Check sheet for the drawn part. Datum: minimum x, y, z corner. Units: mm. Round coordinates to 2 decimals unless told otherwise and drop trailing zeros. Loops run counter-clockwise (first coordinate to the right, second up) from the corner with the lowest first, then second, coordinate; pieces in that order, holes last. Notation, with made-up numbers: (46, 65.25) -> (105, 65.25) arc R8 cw to (105, 72.25) -> close; hole circle Ø11 at (20.5, 65.25). An arc over 180 degrees is marked (long way). Write item = value, one per line. Start each with the question number.
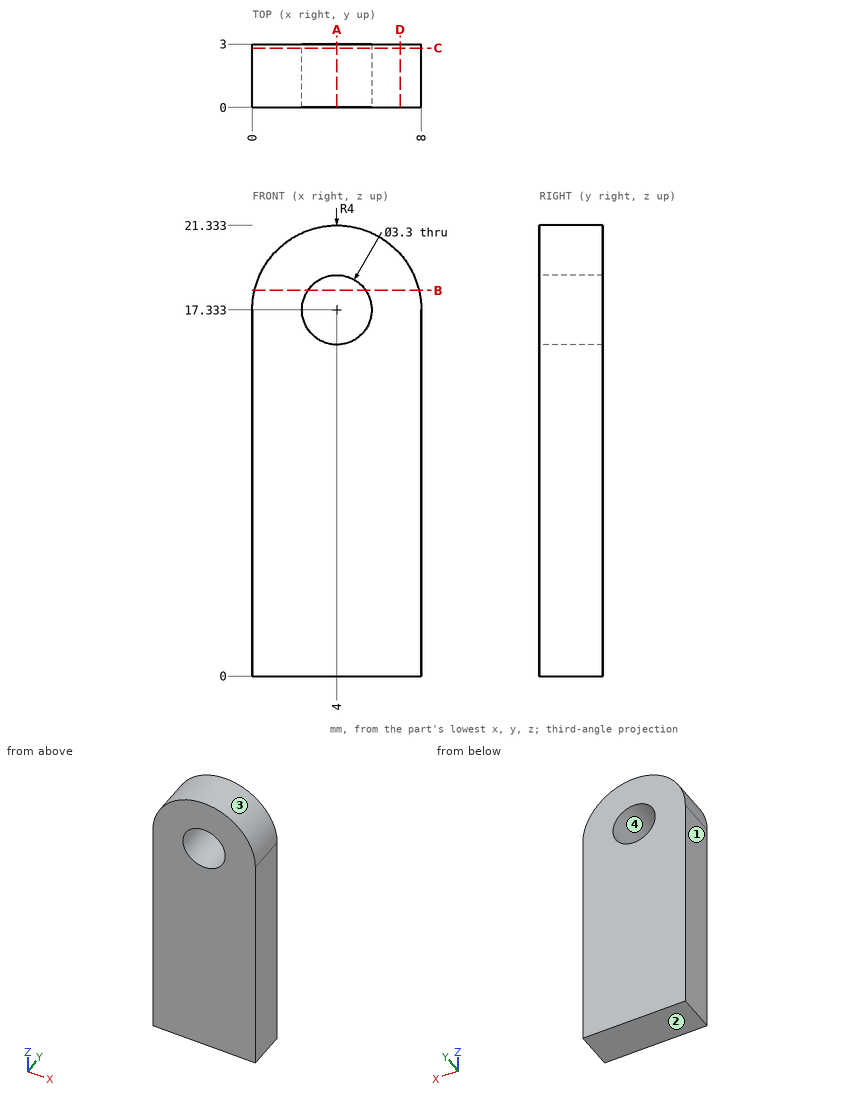
(1) Draft check along Z on the marked faces 1, 2, 3 and 4. Enter one of: +Z half, -Z half, draft (parallel to the pull), parting line (faces both ways), or undercut.
(2) Section check C-C on y = 2.8. Enter the section's corners in (x, z).
(3) Scan lines: line 1 (Z direction, x = 4, y = 2); line 2 (Z direction, x = 5, y = 2.8) (1 decimal); line 3 (X direction, y = 2.65, z = 16.5). Record each from-to range of solid material in increasing order. Write a range as [from, to].
(4) Depth check by flat-ended pin: pin 1 Ø1.5 at (x, y) = (3, 2.5) entering from +Z (3 decimals); pin 2 Ø2 at (x, z) = (6, 4.5) entering from -Y; pin 3 Ø1 at (x, y) = (7, 0.5) entering from +Z; pin 4 Ø3 at (x, z) = (4, 17.33) entering from +Y. Enter the tip coordinate at first touch or a pass-through.
(5) Section check D-D on x = 7. Enter the section's corners in (y, z).
(6) Section check B-B on z = 18.25. Enter the section's corners in (x, y).
(7) Section check A-A on x = 4. Enter the section's corners in (y, z), then the cut area to 3 significant figures.
Computed values:
q1.face_1 = draft
q1.face_2 = -Z half
q1.face_3 = +Z half
q1.face_4 = undercut
q2.outline = (0, 0) -> (8, 0) -> (8, 17.33) arc R4 ccw to (0, 17.33) -> close; hole circle Ø3.3 at (4, 17.33)
q3.line_1 = [0, 15.68], [18.98, 21.33]
q3.line_2 = [0, 16], [18.6, 21.2]
q3.line_3 = [0, 2.58], [5.42, 8]
q4.pin_1 = 21.325
q4.pin_2 = 0
q4.pin_3 = 20.46
q4.pin_4 = through
q5.outline = (0, 0) -> (3, 0) -> (3, 19.98) -> (0, 19.98) -> close
q6.outline = (0.11, 0) -> (2.63, 0) -> (2.63, 3) -> (0.11, 3) -> close; (5.37, 0) -> (7.89, 0) -> (7.89, 3) -> (5.37, 3) -> close
q7.outline = (0, 0) -> (3, 0) -> (3, 15.68) -> (0, 15.68) -> close; (0, 18.98) -> (3, 18.98) -> (3, 21.33) -> (0, 21.33) -> close
q7.area = 54.1 mm²
